Check sheet for the modelled part. Datum: model origin and axes. Units: mm. A direction names the side the tool comes from. Give positions to 0.01 mm unless a question says otherwise; leave off trailing zeros. Loops run counter-clockwise (first coordinate to the right, second up) from the corner with the lowest first, then second, coordinate; pieces in that order, holes last.
```python
from build123d import *

# Parameters (mm, degrees)
SKETCH1_W           = 60
SKETCH1_H           = 35
BOSS_EXTRUDE1_DEPTH = 18
SKETCH2_R           = 3.075
CUT_EXTRUDE1_DEPTH  = 18
SKETCH3_R           = 1.45
SKETCH3_W           = 36.5
SKETCH3_H           = 26
CUT_EXTRUDE2_DEPTH  = 11
SKETCH4_R           = 2.975
BOSS_EXTRUDE2_DEPTH = 11.8
SKETCH6_R           = 1
CUT_EXTRUDE3_DEPTH  = 5.8
SKETCH8_R           = 1
CUT_EXTRUDE4_DEPTH  = 5.8
FILLET2_R           = 0.5


with BuildPart() as part:
    # Sketch1 → Boss-Extrude1 (new body)
    with BuildSketch(Plane.XY):
        with Locations((30, 17.5)):
            Rectangle(SKETCH1_W, SKETCH1_H)
    extrude(amount=BOSS_EXTRUDE1_DEPTH)

    # Sketch2 → Cut-Extrude1 (cut)
    with BuildSketch(Plane.XY.offset(18)):
        with Locations((11.25, 26)):
            Circle(SKETCH2_R)
        with Locations((11.25, 9)):
            Circle(SKETCH2_R)
    extrude(amount=-CUT_EXTRUDE1_DEPTH, mode=Mode.SUBTRACT)

    # Sketch3 → Cut-Extrude2 (cut)
    with BuildSketch(Plane.XY.offset(18)):
        with Locations((3, 32)):
            Circle(SKETCH3_R)
        with Locations((57, 32)):
            Circle(SKETCH3_R)
        with Locations((57, 3)):
            Circle(SKETCH3_R)
        with Locations((3, 3)):
            Circle(SKETCH3_R)
        with Locations((36.25, 17.5)):
            Rectangle(SKETCH3_W, SKETCH3_H)
    extrude(amount=-CUT_EXTRUDE2_DEPTH, mode=Mode.SUBTRACT)

    # Sketch4 → Boss-Extrude2 (add)
    with BuildSketch(Plane.XY.offset(7)):
        with Locations(Location((25, 17.5, 0), (0, 0, 180))):
            Circle(SKETCH4_R)
        with Locations(Location((36.25, 15, 0), (0, 0, 180))):
            Circle(SKETCH4_R)
        with Locations(Location((47.5, 17.5, 0), (0, 0, 180))):
            Circle(SKETCH4_R)
    extrude(amount=BOSS_EXTRUDE2_DEPTH)

    # Sketch6 → Cut-Extrude3 (cut)
    with BuildSketch(Plane(origin=(60, 0, 0), x_dir=(0, 0, -1), z_dir=(1, 0, 0))):
        with Locations((-9, 20.475)):
            Circle(SKETCH6_R)
    extrude(amount=-CUT_EXTRUDE3_DEPTH, mode=Mode.SUBTRACT)

    # Sketch8 → Cut-Extrude4 (cut)
    with BuildSketch(Plane.XZ):
        with Locations(Location((22.025, 9, 0), (0, 0, 270))):
            Circle(SKETCH8_R)
    extrude(amount=-CUT_EXTRUDE4_DEPTH, mode=Mode.SUBTRACT)

    # Fillet2
    fillet2_edges = [part.edges().sort_by_distance(p)[0] for p in [
        (54.5, 20.475, 10),
        (60, 20.475, 10),
        (22.025, 4.5, 10),
        (22.025, 0, 10),
    ]]
    fillet(fillet2_edges, radius=FILLET2_R)


solid = part.part
```
(1) Section check B-B on x = 11.25. Record the boundary of the cut face in (y, z) (3 decimals), plus the area to 3 significant figures.
(2) Material ranges on line 1 (Y direction, x = 11.5, z = 14); line 2 (Y direction, x = 3, z = 10.5); line 3 (X direction, y = 3.3, z = 9) (3 decimals), recorded low to high.
(3) Access from +Z, -Z, +X, -X, +Y, -Y to the whole of each face (thin tool, end or side, straight path). Record for faces 4 (the face through (8.81, 7.13, 9.13)), 5 (the face through (36, 21, 7)), 6 (the face through (57.282, 19.867, 9.794)).
(4) Section check A-A on z = 9. Give the number of separate pieces and of enclosed holes in the cut face, plus the area to 3 significant figures.
(5) Release check for a two-part mould opening along Y. For faces 1 (the face through (60, 17, 9)), 2 (the face through (54.5, 17, 13)), 3 (the face through (30, 0, 9)) record: pulls with the +Y half, pulls with the -Y half, needs draft (parallel to the pull), parting line crosses it, or undercut.
(6) Section check D-D on y = 26. Record the boundary of the cut face in (x, z) (3 decimals).
(7) Gauge pin test, flat ends, axial feed: pin 1 Ø2.5 at (x, y) = (57, 3) entering from +Z; pin 2 Ø5 at (x, y) = (11.25, 26) entering from -Z; pin 3 Ø3 at (x, y) = (56.5, 32) entering from +Z; pin 4 Ø1.2 at (x, z) = (22.025, 9) entering from -Y. Record the tip position at first contact, or that the pin passes through.
Computed values:
1. outline: (0, 0) - (5.925, 0) - (5.925, 18) - (0, 18) - close; (12.075, 0) - (22.925, 0) - (22.925, 18) - (12.075, 18) - close; (29.075, 0) - (35, 0) - (35, 18) - (29.075, 18) - close
1. area: 409 mm2
2. line 1: y = 0 to 5.94, 12.06 to 22.94, 29.06 to 35
2. line 2: y = 0 to 1.55, 4.45 to 30.55, 33.45 to 35
2. line 3: x = 0 to 1.581, 4.419 to 21.025, 23.025 to 55.581, 58.419 to 60
3. face 4: +Z, -Z
3. face 5: +Z
3. face 6: +X
4. separate pieces: 5
4. enclosed holes: 6
4. area: 1,130 mm2
5. face 1: needs draft
5. face 2: undercut
5. face 3: pulls with the -Y half
6. outline: (0, 0) - (8.175, 0) - (8.175, 18) - (0, 18) - close; (14.325, 0) - (60, 0) - (60, 18) - (54.5, 18) - (54.5, 7) - (18, 7) - (18, 18) - (14.325, 18) - close
7. pin 1: stops at z = 7
7. pin 2: passes through
7. pin 3: stops at z = 18
7. pin 4: stops at y = 15.71
